Design review of the part built by this model. Coordinates are the model's own, in mm. A direction names the side the tool comes from. Give positions to 0.01 mm unless a question says otherwise; leave off trailing zeros. Loops run counter-clockwise (first coordinate to the right, second up) from the corner with the lowest first, then second, coordinate; pieces in that order, holes last. Notation, with made-up numbers: (52.5, 81) -> (100.5, 81) arc R17 cw to (100.5, 93) -> close; hole circle Ø11 at (33.5, -8.5). An arc over 180 degrees is marked (long way). Use a Markdown table: item, result. Add a question column.
1. Add section B-B (z = 49). State the section outline as (x, y) points.
2. Draft analysis for pull direction Y (two halves, no side actions). For faces 1 (the flat face through (2.5, -1, 32)), 2 (the flat face through (1, -0.76, 78)), 3 (the flat face through (1, -50, 15)), 4 (the flat face through (1, 44.062, 2)), state which applies: pulls with the +Y half, pulls with the -Y half, needs draft (parallel to the pull), parting line crosses it, or undercut.
3. For faces 5 (the flat face through (1, -45.562, 2)), 6 (the flat face through (1, 0.74, 78)), 7 (the flat face through (1, -31, 29.988)), list the 3-axis set-ups (+Z, -Z, +X, -X, +Y, -Y) from which the entire face can be reached by the end or side of a thin tool; tool diameter is ignored.
4. To check wall thickness, follow line 1 (Y direction, x = 1.7, z = 4.5); line 2 (Z direction, x = 1.9, y = 1.5); line 3 (Z direction, x = 2.25, y = -23). State the ranges of each line that lie inside material, in increasing order.
5. For pin 1 Ø0.8 at (x, y) = (1.5, 34) entering from +Z; pin 2 Ø0.8 at (x, z) = (1, 74.5) entering from -Y; pin 3 Ø8 at (y, z) = (0, 33) entering from -X; pin 4 Ø1.2 at (x, y) = (1.5, -44.5) entering from -Z, all flat-tipped, find the tip position at first contact; note any pin that passes through.
6. Add section A-A (y = -40). State the section outline as (x, z) points.
```python
from build123d import *

# Parameters (mm, degrees)
F1_DEPTH = 2.5


# Not quite as in the source:
# - a feature names something its author has since deleted; it is built from what else it names


with BuildPart() as f1:
    # F0 (on Right) → F1 (new body)
    with BuildSketch(Plane.YZ):
        Polygon((45.5622866154, 0), (50, -0.0115907192), (50, 29.9884092808), (13.482012786, 29.9884092808), (13.482012786, 79.9884092808), (0.7398080197, 79.910288877), (0.7398080197, 75.2277448773), (2.2398080197, 75.2277448773), (2.2398080197, 73.7277448773), (0.7398080197, 73.7277448773), (0.7398080197, 72.2277448773), (-0.7601919803, 72.2277448773), (-0.7601919803, 73.7277448773), (-2.2601919803, 73.7277448773), (-2.2601919803, 75.2277448773), (-0.7601919803, 75.2277448773), (-0.7601919803, 79.9100687942), (-13.482012786, 79.9884092808), (-13.482012786, 29.9884092808), (-50, 29.9884092808), (-50, -0.0115907192), (-45.5622866154, 0), (-45.5622866154, 3.739590158), (-47.0622866154, 3.739590158), (-47.0622866154, 5.239590158), (-45.5622866154, 5.239590158), (-45.5622866154, 6.739590158), (-44.0622866154, 6.739590158), (-44.0622866154, 5.239590158), (-42.5622866154, 5.239590158), (-42.5622866154, 3.739590158), (-44.0622866154, 3.739590158), (-44.0622866154, 0), (0, 0), (44.0622866154, 0), (44.0622866154, 3.739590158), (42.5622866154, 3.739590158), (42.5622866154, 5.239590158), (44.0622866154, 5.239590158), (44.0622866154, 6.739590158), (45.5622866154, 6.739590158), (45.5622866154, 5.239590158), (47.0622866154, 5.239590158), (47.0622866154, 3.739590158), (45.5622866154, 3.739590158), align=None)
    extrude(amount=F1_DEPTH)


solid = f1.part
```
Taken from the geometry:
| question | item | result |
|---|---|---|
| 1 | outline | (0, -13.48) -> (2.5, -13.48) -> (2.5, 13.48) -> (0, 13.48) -> close |
| 2 | face 1 | needs draft |
| 2 | face 2 | undercut |
| 2 | face 3 | pulls with the -Y half |
| 2 | face 4 | undercut |
| 3 | face 5 | -Z, +X, -X |
| 3 | face 6 | +Z, +X, -X |
| 3 | face 7 | +Z, +X, -X, -Y |
| 4 | line 1 | y = -50 to -47.06, -42.56 to 42.56, 47.06 to 50 |
| 4 | line 2 | z = 0 to 73.73, 75.23 to 79.91 |
| 4 | line 3 | z = 0 to 29.99 |
| 5 | pin 1 | stops at z = 29.99 |
| 5 | pin 2 | stops at y = -13.48 |
| 5 | pin 3 | stops at x = 0 |
| 5 | pin 4 | stops at z = 0 |
| 6 | outline | (0, 0) -> (2.5, 0) -> (2.5, 29.99) -> (0, 29.99) -> close |
